Design review of the part built by this model. Coordinates are the model's own, in mm. A direction names the side the tool comes from. Round coordinates to 2 decimals unless told otherwise and drop trailing zeros. Order: outer loops, then holes, each group sorted by start corner. A loop starts at its lowest first (then second) coordinate and runs counter-clockwise, first axis right, second up. Notation, with made-up numbers: M 78.25,79.5 L 111.25,79.5 A35 cw 111.25,114.5 Z; hole C -22,39.5 d4. An arc over 180 degrees is marked long. Use a Markdown table: item, result. Add a question column.
(1) Take a section at B-B (y = -37.5). Write out the cut boundary in (x, z), then the cut area to 3 significant figures.
(2) Take a section at C-C (x = -6.5). Write out the cut boundary in (y, z), then the cut area to 4 significant figures.
(3) To check wall thickness, follow probe 1 along X at (y, z) = (-52, 2); probe 2 along Z at (x, y) = (-16, -39.5); probe 3 along Z at (x, y) = (-25.5, -48). State the ranges of each line that lie inside material, in increasing order. Write a range as from..to.
(4) For pin 1 (3 mm diameter, centred on y = -48, z = -2, fed in from +X); pin 2 (5 mm diameter, centred on x = -17, z = -3.5, fed in from -Y); pin 3 (2 mm diameter, centred on y = -38, z = -4, fed in from -X); pin 4 (0.8 mm diameter, centred on x = -16, z = 2, fed in from +Y), all flat-tipped, find the tip position at first contact; note any pin that passes through.
(5) Take a section at D-D (y = -50.5). Write out the cut boundary in (x, z).
(6) Machinability: for faces 1 (the face through (-15, -59.157, 2)), 2 (the face through (-28.434, -37.376, 0.74)), 3 (the face through (-1.884, -50, 2)), which of the approach directions +Z, -Z, +X, -X, +Y, -Y give a long, thin tool a straight path to every point of the face, cutting with its end or side? Answer none if there is none.
(7) The part is to be moulded in two halves that separate along Y. For faces 4 (the face through (-3, -36.507, 1)), 5 (the face through (-15, -35.507, 1)), 6 (the face through (-15, -39, 1.5)), 7 (the face through (-15, -63.507, 1)), say which applies: released by +Y, released by -Y, zero draft, split by the parting line, or undercut.
(8) Take a section at A-A (z = 1). Write out the cut boundary in (x, y).
```python
from build123d import *

# Parameters (mm, degrees)
EXTRUDE_1_DEPTH = 1.5
SKETCH_2_W      = 26.6
SKETCH_2_H      = 19.3
EXTRUDE_2_DEPTH = 1.5
SKETCH_3_W      = 10
SKETCH_3_H      = 2.5
EXTRUDE_3_DEPTH = 10


with BuildPart() as part:
    # 草圖1 → 填料-伸長1 (new body)
    with BuildSketch(Plane.XY):
        Polygon((-28.934480155, -35.507444045), (-1.434480155, -35.507444045), (-0.934480155, -36.007444045), (-0.934480155, -63.007444045), (-1.434480155, -63.507444045), (-28.934480155, -63.507444045), (-29.434480155, -63.007444045), (-29.434480155, -36.007444045), align=None)
        with BuildLine():
            Line((-4.084480155, -36.507444045), (-2.784480155, -36.507444045))
            ThreePointArc((-2.784480155, -36.507444045), (-1.934480155, -37.357444045), (-2.784480155, -38.207444045))
            Line((-2.784480155, -38.207444045), (-4.084480155, -38.207444045))
            ThreePointArc((-4.084480155, -38.207444045), (-4.934480155, -37.357444045), (-4.084480155, -36.507444045))
        make_face(mode=Mode.SUBTRACT)
        with BuildLine():
            Line((-27.584480155, -36.507444045), (-26.284480155, -36.507444045))
            ThreePointArc((-26.284480155, -36.507444045), (-25.434480155, -37.357444045), (-26.284480155, -38.207444045))
            Line((-26.284480155, -38.207444045), (-27.584480155, -38.207444045))
            ThreePointArc((-27.584480155, -38.207444045), (-28.434480155, -37.357444045), (-27.584480155, -36.507444045))
        make_face(mode=Mode.SUBTRACT)
        with BuildLine():
            Line((-27.584480155, -60.807444045), (-26.284480155, -60.807444045))
            ThreePointArc((-26.284480155, -60.807444045), (-25.434480155, -61.657444045), (-26.284480155, -62.507444045))
            Line((-26.284480155, -62.507444045), (-27.584480155, -62.507444045))
            ThreePointArc((-27.584480155, -62.507444045), (-28.434480155, -61.657444045), (-27.584480155, -60.807444045))
        make_face(mode=Mode.SUBTRACT)
        with BuildLine():
            Line((-4.084480155, -60.807444045), (-2.784480155, -60.807444045))
            ThreePointArc((-2.784480155, -60.807444045), (-1.934480155, -61.657444045), (-2.784480155, -62.507444045))
            Line((-2.784480155, -62.507444045), (-4.084480155, -62.507444045))
            ThreePointArc((-4.084480155, -62.507444045), (-4.934480155, -61.657444045), (-4.084480155, -60.807444045))
        make_face(mode=Mode.SUBTRACT)
    extrude(amount=EXTRUDE_1_DEPTH)

    # 草圖2 → 填料-伸長2 (add)
    with BuildSketch(Plane.XY.offset(1.5)):
        with Locations((-15.184480155, -49.507444045)):
            Rectangle(SKETCH_2_W, SKETCH_2_H)
    extrude(amount=EXTRUDE_2_DEPTH)

    # 草圖3 → 填料-伸長3 (add)
    with BuildSketch(Plane(origin=(0, 0, 0), x_dir=(-1, 0, 0), z_dir=(0, 0, -1))):
        with Locations((15.184480155, -37.257444045)):
            Rectangle(SKETCH_3_W, SKETCH_3_H)
    extrude(amount=EXTRUDE_3_DEPTH)


solid = part.part
```
Verdict:
| question | item | result |
|---|---|---|
| 1 | outline | M -29.43,0 L -28.42,0 L -28.42,1.5 L -29.43,1.5 Z; M -25.45,0 L -20.18,0 L -20.18,-10 L -10.18,-10 L -10.18,0 L -4.92,0 L -4.92,1.5 L -25.45,1.5 Z; M -1.95,0 L -0.93,0 L -0.93,1.5 L -1.95,1.5 Z |
| 1 | area | 134 mm^2 |
| 2 | outline | M -63.51,0 L -35.51,0 L -35.51,1.5 L -39.86,1.5 L -39.86,3 L -59.16,3 L -59.16,1.5 L -63.51,1.5 Z |
| 2 | area | 70.95 mm^2 |
| 3 | probe 1 | x = -28.48..-1.88 |
| 3 | probe 2 | z = 0..1.5 |
| 3 | probe 3 | z = 0..3 |
| 4 | pin 1 | passes through |
| 4 | pin 2 | stops at y = -38.51 |
| 4 | pin 3 | stops at x = -20.18 |
| 4 | pin 4 | stops at y = -39.86 |
| 5 | outline | M -29.43,0 L -0.93,0 L -0.93,1.5 L -1.88,1.5 L -1.88,3 L -28.48,3 L -28.48,1.5 L -29.43,1.5 Z |
| 6 | face 1 | +Z, +X, -X, -Y |
| 6 | face 2 | +Z, -Z |
| 6 | face 3 | +Z, +X, +Y, -Y |
| 7 | face 4 | undercut |
| 7 | face 5 | released by +Y |
| 7 | face 6 | zero draft |
| 7 | face 7 | released by -Y |
| 8 | outline | M -29.43,-63.01 L -28.93,-63.51 L -1.43,-63.51 L -0.93,-63.01 L -0.93,-36.01 L -1.43,-35.51 L -28.93,-35.51 L -29.43,-36.01 Z; hole M -27.58,-62.51 L -26.28,-62.51 A0.85 ccw -26.28,-60.81 L -27.58,-60.81 A0.85 ccw Z; hole M -27.58,-38.21 L -26.28,-38.21 A0.85 ccw -26.28,-36.51 L -27.58,-36.51 A0.85 ccw Z; hole M -4.08,-62.51 L -2.78,-62.51 A0.85 ccw -2.78,-60.81 L -4.08,-60.81 A0.85 ccw Z; hole M -4.08,-38.21 L -2.78,-38.21 A0.85 ccw -2.78,-36.51 L -4.08,-36.51 A0.85 ccw Z |
